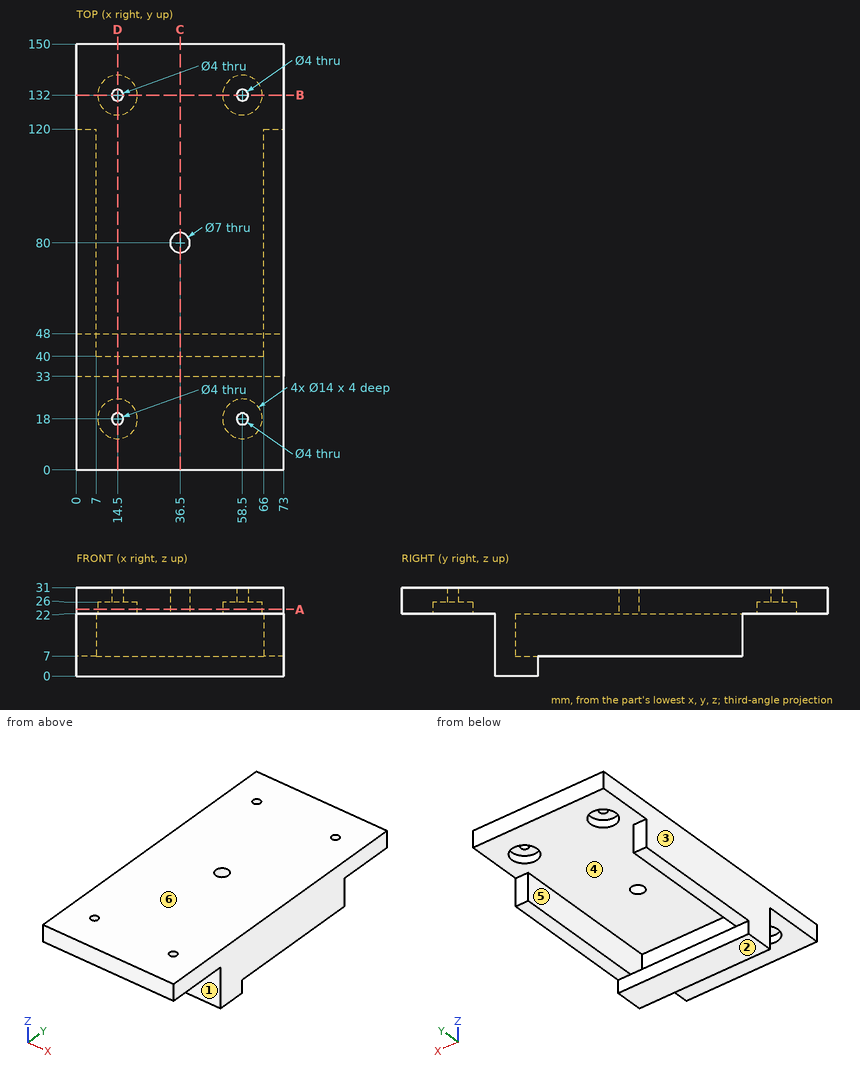
The drawing under review shows one solid part. Ordinate dimensions are in mm from its lowest x, y, z. A direction names the side the tool comes from. Coordinates: 2 decimals unless noted, no trailing zeros. Write each loop counter-clockwise with the first axis right and the second up, starting at its lowest first coordinate (ties: lowest second). Pieces come first, ordered by that corner, then holes. Notation, with made-up numbers: (76.5, 21) - (99.5, 21) arc R28 cw to (99.5, 49) - close; hole circle Ø5 at (-7.5, 51). An arc over 180 degrees is marked (long way). Answer as CSV lines item,"result".
(1) Clearance check with flat-ended pins moving along their axes: pin 1 Ø7.5 at (x, y) = (69, 95.5) entering from -Z; pin 2 Ø1.5 at (x, z) = (55, 4) entering from +Y; pin 3 Ø3.5 at (x, z) = (4, 14) entering from +Y; pin 4 Ø3.5 at (x, y) = (58.5, 132) entering from -Z. State where each tip first meets the part, or that it passes through.
Data:
pin 1,"stops at z = 7"
pin 2,"stops at y = 48"
pin 3,"stops at y = 120"
pin 4,"passes through"
(2) We need section D-D (x = 14.5). Give the boundary of the cut face in (y, z), plus the area to 3 significant figures.
Data:
outline,"(0, 22) - (11, 22) - (11, 26) - (16, 26) - (16, 31) - (0, 31) - close; (20, 26) - (25, 26) - (25, 22) - (33, 22) - (33, 0) - (48, 0) - (48, 7) - (40, 7) - (40, 22) - (125, 22) - (125, 26) - (130, 26) - (130, 31) - (20, 31) - close; (134, 26) - (139, 26) - (139, 22) - (150, 22) - (150, 31) - (134, 31) - close"
area,"1,410 mm2"
(3) Tool access review of the marked faces 1 and 2: name each direction out of +Z, -Z, +X, -X, +Y, -Y from which nothing blocks a thin tool from reaching the whole face with its end or side.
Data:
face 1,"-Z, +X, -X, -Y"
face 2,"-Z, +X, -X, +Y, -Y"
(4) We need section B-B (y = 132). Give the boundary of the cut face in (x, z).
Data:
outline,"(0, 22) - (7.5, 22) - (7.5, 26) - (12.5, 26) - (12.5, 31) - (0, 31) - close; (16.5, 26) - (21.5, 26) - (21.5, 22) - (51.5, 22) - (51.5, 26) - (56.5, 26) - (56.5, 31) - (16.5, 31) - close; (60.5, 26) - (65.5, 26) - (65.5, 22) - (73, 22) - (73, 31) - (60.5, 31) - close"
(5) We need section C-C (x = 36.5). Give the boundary of the cut face in (y, z).
Data:
outline,"(0, 22) - (33, 22) - (33, 0) - (48, 0) - (48, 7) - (40, 7) - (40, 22) - (76.5, 22) - (76.5, 31) - (0, 31) - close; (83.5, 22) - (150, 22) - (150, 31) - (83.5, 31) - close"
(6) For line 1 along Y through (x, z) = (14.5, 22.8); line 2 along Y through (x, z) = (58.5, 29.9); line 3 along X through (y, z) = (46, 9), list the stretches that pass through material, from the lowest coordinate up. Write a range as [from, to].
Data:
line 1,"y = [0, 11], [25, 125], [139, 150]"
line 2,"y = [0, 16], [20, 130], [134, 150]"
line 3,"x = [0, 7], [66, 73]"
(7) We need section A-A (z = 23.5). Give the boundary of the cut face in (x, y), plus the area to 3 significant figures.
Data:
outline,"(0, 0) - (73, 0) - (73, 150) - (0, 150) - close; hole circle Ø14 at (14.5, 18); hole circle Ø14 at (14.5, 132); hole circle Ø7 at (36.5, 80); hole circle Ø14 at (58.5, 18); hole circle Ø14 at (58.5, 132)"
area,"10,300 mm2"
(8) Mouldability with a two-part tool opening along X and no side actions: class the marked faces 3, 4, 5 and 6 as pulls with the +X half, pulls with the -X half, needs draft (parallel to the pull), parting line crosses it, or undercut.
Data:
face 3,"pulls with the -X half"
face 4,"undercut"
face 5,"undercut"
face 6,"needs draft"
